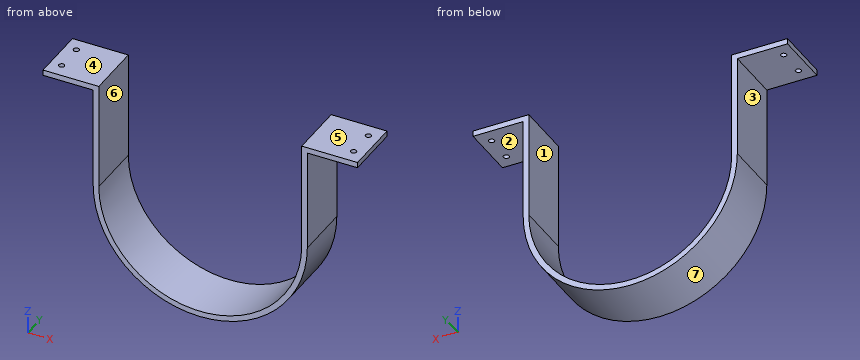
```python
from build123d import *

# Parameters (mm, degrees)
BOSS_EXTRUDE1_DEPTH = 31.75
SKETCH3_R           = 3.175
CUT_EXTRUDE2_DEPTH  = 6.35


with BuildPart() as part:
    # Sketch1 → Boss-Extrude1 (new, symmetric)
    with BuildSketch(Plane(origin=(0, 0, 0), x_dir=(1, 0, 0), z_dir=(0, 1, 0))):
        with BuildLine():
            Line((-114.7, -121.05), (-114.7, 0))
            ThreePointArc((-114.7, 0), (0, 114.7), (114.7, 0))
            Line((114.7, 0), (114.7, -121.05))
            Line((114.7, -121.05), (177.8, -121.05))
            Line((177.8, -121.05), (177.8, -114.7))
            Line((177.8, -114.7), (121.05, -114.7))
            Line((121.05, -114.7), (121.05, 0))
            ThreePointArc((121.05, 0), (0, 121.05), (-121.05, 0))
            Line((-121.05, 0), (-121.05, -12.7))
            Line((-121.05, -12.7), (-121.05, -114.7))
            Line((-121.05, -114.7), (-177.8, -114.7))
            Line((-177.8, -114.7), (-177.8, -121.05))
            Line((-177.8, -121.05), (-114.7, -121.05))
        make_face()
    extrude(amount=BOSS_EXTRUDE1_DEPTH, both=True)

    # Sketch3 → Cut-Extrude2 (cut)
    with BuildSketch(Plane.XY.offset(121.05)):
        with Locations((-165.1, 15.875)):
            Circle(SKETCH3_R)
        with Locations((-165.1, -15.875)):
            Circle(SKETCH3_R)
        with Locations((165.1, -15.875)):
            Circle(SKETCH3_R)
        with Locations((165.1, 15.875)):
            Circle(SKETCH3_R)
    extrude(amount=-CUT_EXTRUDE2_DEPTH, mode=Mode.SUBTRACT)


solid = part.part
```
Verification items for the finished model (mm, model axes). Face numbers are marked on the shaded views. A direction names the side the tool comes from. Coordinates: 2 decimals unless noted, no trailing zeros. Loops run counter-clockwise (first coordinate to the right, second up) from the corner with the lowest first, then second, coordinate; pieces in that order, holes last. Notation, with made-up numbers: (10.25, 41) -> (54.25, 41) arc R34 cw to (54.25, 72) -> close; hole circle Ø1 at (45.5, -32.5). An arc over 180 degrees is marked (long way). Answer in a Markdown table with one row per item. Add a question column.
1. Section check C-C, the plane x = -132.5. Enter the section's corners in (y, z).
2. Depth check by flat-ended pin: P1, Ø4, axis at x = -20, y = 23.5, coming from the +Z side; P2, Ø19, axis at y = 12.5, z = 65.5, coming from the +X side; P3, Ø2, axis at x = -18.5, y = -19.5, coming from the -Z side; P4, Ø8.5, axis at x = 165.1, y = -15.875, coming from the +Z side. Enter the tip coordinate at first touch or a pass-through.
3. Section check A-A, the plane z = 93. Enter the section's corners in (x, y), then the cut area to 3 significant figures.
4. Section check D-D, the plane x = -24.5. Enter the section's corners in (y, z).
5. Draft check along X on the marked faces 5, 6 and 7. Enter one of: +X half, -X half, draft (parallel to the pull), parting line (faces both ways), or undercut.
6. Material ranges on probe 1 along Y at (x, z) = (-165.1, 116.25); probe 2 along X at (y, z) = (-21.5, 108); probe 3 along Z at (x, y) = (-139, 17), recorded low to high. Write a range as [from, to].
7. Section check B-B, the plane z = -66. Enter the section's corners in (x, y).
8. Access from +Z, -Z, +X, -X, +Y, -Y to the whole of each face (thin tool, end or side, straight path). Record for the marked faces 1, 2, 3 and 4.
Derived:
| question | item | result |
|---|---|---|
| 1 | outline | (-31.75, 114.7) -> (31.75, 114.7) -> (31.75, 121.05) -> (-31.75, 121.05) -> close |
| 2 | P1 | stops at z = -112.57 |
| 2 | P2 | stops at x = 121.05 |
| 2 | P3 | stops at z = -119.78 |
| 2 | P4 | stops at z = 121.05 |
| 3 | outline | (-121.05, -31.75) -> (-114.7, -31.75) -> (-114.7, 31.75) -> (-121.05, 31.75) -> close; (114.7, -31.75) -> (121.05, -31.75) -> (121.05, 31.75) -> (114.7, 31.75) -> close |
| 3 | area | 806 mm² |
| 4 | outline | (-31.75, -118.54) -> (31.75, -118.54) -> (31.75, -112.05) -> (-31.75, -112.05) -> close |
| 5 | face 5 | draft |
| 5 | face 6 | undercut |
| 5 | face 7 | parting line |
| 6 | probe 1 | y = [-31.75, -19.05], [-12.7, 12.7], [19.05, 31.75] |
| 6 | probe 2 | x = [-121.05, -114.7], [114.7, 121.05] |
| 6 | probe 3 | z = [114.7, 121.05] |
| 7 | outline | (-101.47, -31.75) -> (-93.81, -31.75) -> (-93.81, 31.75) -> (-101.47, 31.75) -> close; (93.81, -31.75) -> (101.47, -31.75) -> (101.47, 31.75) -> (93.81, 31.75) -> close |
| 8 | face 1 | +Z, +Y, -Y |
| 8 | face 2 | -Z, +X, +Y, -Y |
| 8 | face 3 | -Z, -X, +Y, -Y |
| 8 | face 4 | +Z, +X, -X, +Y, -Y |
